Job drawing, mm, ordinate dimensions from the low corner. One solid piece. Give positions to 0.01 mm unless a question says otherwise; leave off trailing zeros. Loops run counter-clockwise (first coordinate to the right, second up) from the corner with the lowest first, then second, coordinate; pieces in that order, holes last. Notation, with made-up numbers: (4.5, -12.5) -> (28.5, -12.5) arc R13 ccw to (28.5, 5.5) -> close; hole circle Ø1 at (12, 35.25). An arc over 180 degrees is marked (long way). Use one line per item in the form item = value.
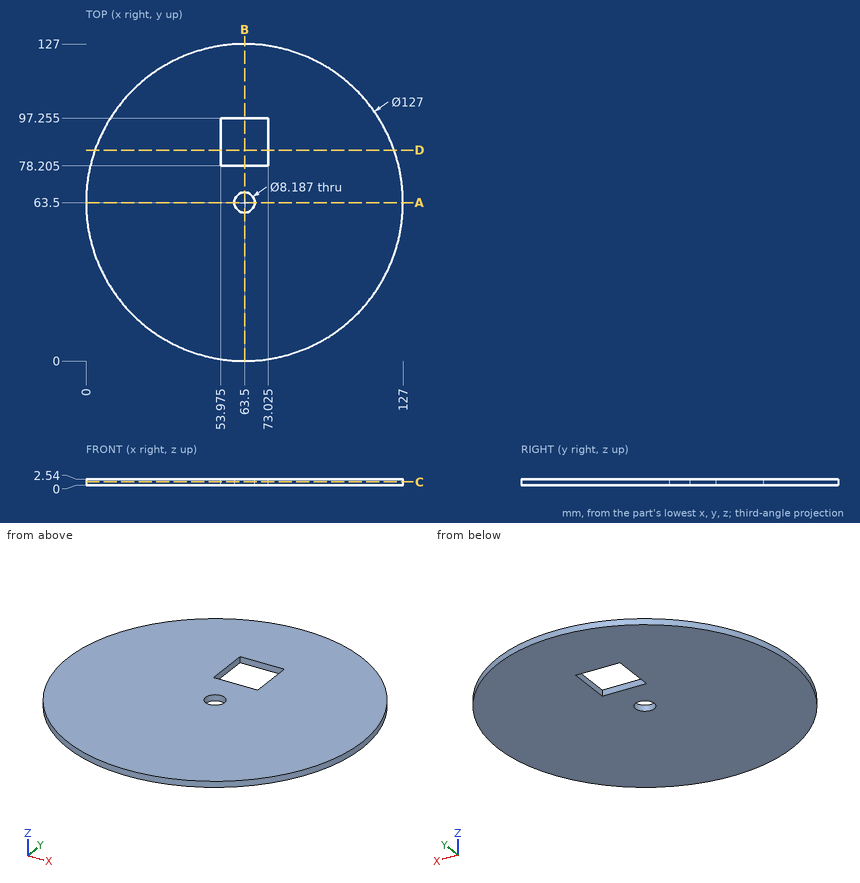
1. Cut at C-C, the plane z = 1.4. Write the cut outline in (x, y) (1 decimal), then the cut area to 3 significant figures.
Result sheet:
outline = circle Ø127 at (63.5, 63.5); hole (54, 78.2) -> (73, 78.2) -> (73, 97.3) -> (54, 97.3) -> close; hole circle Ø8.2 at (63.5, 63.5)
area = 12,300 mm^2
2. Drill centre lines: line 1 (Y direction, x = 63, z = 2.05) (1 decimal); line 2 (X direction, y = 83.5, z = 2.05) (1 decimal); line 3 (Y direction, x = 72, z = 1.3) (1 decimal). Where is each one in solid material? Low to high.
Result sheet:
line_1 = 0 to 59.4, 67.6 to 78.2, 97.3 to 127
line_2 = 3.2 to 54, 73 to 123.8
line_3 = 0.6 to 78.2, 97.3 to 126.4
3. Drop a flat-ended pin along its axis: P1, Ø1.5, axis at x = 70.5, y = 23.5, coming from the -Z side. Give the stop position or say it passes through.
Result sheet:
P1 = 0
4. Cut at D-D, the plane y = 84.5. Write the cut outline in (x, z) (1 decimal), then the cut area to 3 significant figures.
Result sheet:
outline = (3.6, 0) -> (54, 0) -> (54, 2.5) -> (3.6, 2.5) -> close; (73, 0) -> (123.4, 0) -> (123.4, 2.5) -> (73, 2.5) -> close
area = 256 mm^2
5. Cut at A-A, the plane y = 63.5. Write the cut outline in (x, z), then the cut area to 3 significant figures.
Result sheet:
outline = (0, 0) -> (59.41, 0) -> (59.41, 2.54) -> (0, 2.54) -> close; (67.59, 0) -> (127, 0) -> (127, 2.54) -> (67.59, 2.54) -> close
area = 302 mm^2
6. Cut at B-B, the plane x = 63.5. Write the cut outline in (y, z) (1 decimal).
Result sheet:
outline = (0, 0) -> (59.4, 0) -> (59.4, 2.5) -> (0, 2.5) -> close; (67.6, 0) -> (78.2, 0) -> (78.2, 2.5) -> (67.6, 2.5) -> close; (97.3, 0) -> (127, 0) -> (127, 2.5) -> (97.3, 2.5) -> close
